from build123d import *

# Parameters (mm, degrees)
SKETCH2_R           = 50
SKETCH2_R_2         = 2
BOSS_EXTRUDE1_DEPTH = 10
SKETCH3_R           = 21.25
SKETCH3_R_2         = 1.75
SKETCH3_R_3         = 10
CUT_EXTRUDE1_DEPTH  = 5
SKETCH3_2_R         = 1.75
CUT_EXTRUDE2_DEPTH  = 75.1479844
SKETCH3_3_R         = 10
CUT_EXTRUDE3_DEPTH  = 75.1479844


with BuildPart() as part:
    # Sketch2 → Boss-Extrude1 (new body)
    # profile 1 of 5: a face of its own
    with BuildSketch(Plane.XY):
        Circle(SKETCH2_R)
        with BuildLine():
            ThreePointArc((-21.767766953, 18.232233047), (-18.232233047, 18.232233047), (-18.232233047, 21.767766953))
            Line((-18.232233047, 21.767766953), (-28.838834765, 32.374368671))
            ThreePointArc((-28.838834765, 32.374368671), (-32.374368671, 32.374368671), (-32.374368671, 28.838834765))
            Line((-32.374368671, 28.838834765), (-21.767766953, 18.232233047))
        make_face(mode=Mode.SUBTRACT)
        with BuildLine():
            ThreePointArc((-18.232233047, -21.767766953), (-18.232233047, -18.232233047), (-21.767766953, -18.232233047))
            Line((-21.767766953, -18.232233047), (-32.374368671, -28.838834765))
            ThreePointArc((-32.374368671, -28.838834765), (-32.374368671, -32.374368671), (-28.838834765, -32.374368671))
            Line((-28.838834765, -32.374368671), (-18.232233047, -21.767766953))
        make_face(mode=Mode.SUBTRACT)
        with BuildLine():
            ThreePointArc((21.767766953, -18.232233047), (18.232233047, -18.232233047), (18.232233047, -21.767766953))
            Line((18.232233047, -21.767766953), (28.838834765, -32.374368671))
            ThreePointArc((28.838834765, -32.374368671), (32.374368671, -32.374368671), (32.374368671, -28.838834765))
            Line((32.374368671, -28.838834765), (21.767766953, -18.232233047))
        make_face(mode=Mode.SUBTRACT)
        with BuildLine():
            ThreePointArc((18.232233047, 21.767766953), (18.232233047, 18.232233047), (21.767766953, 18.232233047))
            Line((21.767766953, 18.232233047), (32.374368671, 28.838834765))
            ThreePointArc((32.374368671, 28.838834765), (32.374368671, 32.374368671), (28.838834765, 32.374368671))
            Line((28.838834765, 32.374368671), (18.232233047, 21.767766953))
        make_face(mode=Mode.SUBTRACT)
    # profile 2 of 5: a face of its own
    with BuildSketch(Plane.XY):
        with BuildLine():
            ThreePointArc((-47.439646086, 15.794935239), (-34.307195372, 36.373291653), (-12.996869684, 48.281273579))
            ThreePointArc((-12.996869684, 48.281273579), (-23.927789331, 47.432136683), (-34.423317157, 50.602299686))
            ThreePointArc((-34.423317157, 50.602299686), (-48.929401728, 47.913811427), (-49.865534018, 33.190424757))
            ThreePointArc((-49.865534018, 33.190424757), (-46.616230999, 24.776660442), (-47.439646086, 15.794935239))
        make_face()
        with Locations((-39.951533137, 39.951533137)):
            Circle(SKETCH2_R_2, mode=Mode.SUBTRACT)
    # profile 3 of 5: a face of its own
    with BuildSketch(Plane.XY):
        with BuildLine():
            ThreePointArc((15.794935239, 47.439646086), (36.373291653, 34.307195372), (48.281273579, 12.996869684))
            ThreePointArc((48.281273579, 12.996869684), (47.432136683, 23.927789331), (50.602299686, 34.423317157))
            ThreePointArc((50.602299686, 34.423317157), (47.913811427, 48.929401728), (33.190424757, 49.865534018))
            ThreePointArc((33.190424757, 49.865534018), (24.776660442, 46.616230999), (15.794935239, 47.439646086))
        make_face()
        with Locations((39.951533137, 39.951533137)):
            Circle(SKETCH2_R_2, mode=Mode.SUBTRACT)
    # profile 4 of 5: a face of its own
    with BuildSketch(Plane.XY):
        with BuildLine():
            ThreePointArc((49.865534018, -33.190424757), (46.616230999, -24.776660442), (47.439646086, -15.794935239))
            ThreePointArc((47.439646086, -15.794935239), (34.307195372, -36.373291653), (12.996869684, -48.281273579))
            ThreePointArc((12.996869684, -48.281273579), (23.927789331, -47.432136683), (34.423317157, -50.602299686))
            ThreePointArc((34.423317157, -50.602299686), (48.929401728, -47.913811427), (49.865534018, -33.190424757))
        make_face()
        with Locations((39.951533137, -39.951533137)):
            Circle(SKETCH2_R_2, mode=Mode.SUBTRACT)
    # profile 5 of 5: a face of its own
    with BuildSketch(Plane.XY):
        with BuildLine():
            ThreePointArc((-33.190424757, -49.865534018), (-24.776660442, -46.616230999), (-15.794935239, -47.439646086))
            ThreePointArc((-15.794935239, -47.439646086), (-36.373291653, -34.307195372), (-48.281273579, -12.996869684))
            ThreePointArc((-48.281273579, -12.996869684), (-47.432136683, -23.927789331), (-50.602299686, -34.423317157))
            ThreePointArc((-50.602299686, -34.423317157), (-47.913811427, -48.929401728), (-33.190424757, -49.865534018))
        make_face()
        with Locations((-39.951533137, -39.951533137)):
            Circle(SKETCH2_R_2, mode=Mode.SUBTRACT)
    extrude(amount=BOSS_EXTRUDE1_DEPTH)

    # Sketch3 → Cut-Extrude1 (cut)
    with BuildSketch(Plane.XY.offset(10)):
        Circle(SKETCH3_R)
        with Locations((0, 14.5)):
            Circle(SKETCH3_R_2, mode=Mode.SUBTRACT)
        with Locations((12.557368355, -7.25)):
            Circle(SKETCH3_R_2, mode=Mode.SUBTRACT)
        with Locations((-12.557368355, -7.25)):
            Circle(SKETCH3_R_2, mode=Mode.SUBTRACT)
        Circle(SKETCH3_R_3, mode=Mode.SUBTRACT)
    extrude(amount=-CUT_EXTRUDE1_DEPTH, mode=Mode.SUBTRACT)

    # Sketch3_2 → Cut-Extrude2 (cut, through all)
    with BuildSketch(Plane.XY.offset(10)):
        with Locations((0, 14.5)):
            Circle(SKETCH3_2_R)
        with Locations((12.557368355, -7.25)):
            Circle(SKETCH3_2_R)
        with Locations((-12.557368355, -7.25)):
            Circle(SKETCH3_2_R)
    extrude(amount=-CUT_EXTRUDE2_DEPTH, mode=Mode.SUBTRACT)

    # Sketch3_3 → Cut-Extrude3 (cut, through all)
    with BuildSketch(Plane.XY.offset(10)):
        Circle(SKETCH3_3_R)
    extrude(amount=-CUT_EXTRUDE3_DEPTH, mode=Mode.SUBTRACT)


solid = part.part
Can you work these out from the model? Positions are in its coordinate system, mm. A direction names the side the tool comes from. Give positions to 0.01 mm unless a question says otherwise; leave off trailing zeros. Order: outer loops, then holes, each group sorted by start corner. A loop starts at its lowest first (then second) coordinate and runs counter-clockwise, first axis right, second up. Notation, with made-up numbers: M 88.25,21.5 L 134.25,21.5 A20 cw 134.25,51.5 Z; hole C 4.25,59.25 d8. An arc over 180 degrees is marked long. One line per question, with ' | ' between items.
Item 1: We'd pull the mould along X, two halves only. Please class faces 3 (the face through (23.461, -26.997, 4.93)), 4 (the face through (49.972, -1.665, 4.93)), 5 (the face through (-1, -22, 10)), 6 (the face through (-46.634, 24.903, 4.93)): released by +X, released by -X, zero draft, split by the parting line, or undercut.
Answer block:
face 3: undercut | face 4: released by +X | face 5: zero draft | face 6: released by -X
Item 2: I'm going to push flat-ended pins straight in: pin 1 Ø5 at (x, z) = (-23.5, 6.5) entering from +Y; pin 2 Ø3 at (x, y) = (12.56, -7.25) entering from -Z; pin 3 Ø6.5 at (x, y) = (39.95, 39.95) entering from +Z; pin 4 Ø13 at (x, y) = (10, -1) entering from +Z. Where does each tip first touch, or does it pass through?
Answer block:
pin 1: stops at y = 47.73 | pin 2: passes through | pin 3: stops at z = 10 | pin 4: stops at z = 5
Item 3: Suppose I cut it at C-C, the plane y = -26. Write out the boundary of the cut face in (x, z).
Answer block:
outline: M -47.73,0 L -29.54,0 L -29.54,10 L -47.73,10 Z; M -22.46,0 L 22.46,0 L 22.46,10 L -22.46,10 Z; M 29.54,0 L 46.83,0 L 46.83,10 L 29.54,10 Z
Item 4: Please list where these lines run through material, in increasing order: L1, parallel to Y at x = 27.5, z = 1.25; L2, parallel to Y at x = 41.5, z = 5; L3, parallel to X at y = -21, z = 4.
Answer block:
L1: y = -48.04 to -31.04, -23.96 to 23.96, 31.04 to 47.19 | L2: y = -51.85 to -41.22, -38.69 to 38.69, 41.22 to 51.85 | L3: x = -47.26 to -24.54, -17.71 to 17.71, 24.54 to 46.45
Item 5: Suppose I cut it at D-D, the plane z = 2.5. Give the number of separate pieces and of enclosed holes in the cut face, then the cut area to 3 significant figures.
Answer block:
separate pieces: 1 | enclosed holes: 12 | area: 8,910 mm2
Item 6: Suppose I cut it at A-A, the plane y = 0. Write out the boundary of the cut face in (x, z).
Answer block:
outline: M -50,0 L -10,0 L -10,5 L -21.25,5 L -21.25,10 L -50,10 Z; M 10,0 L 50,0 L 50,10 L 21.25,10 L 21.25,5 L 10,5 Z
Item 7: For faces 1 (the face through (23.61, 27.145, 4.93)), 2 (the face through (-49.972, 1.665, 4.93)), which set-ups out of +Z, -Z, +X, -X, +Y, -Y let a thin tool reach every point of the face, with its end or its side?
Answer block:
face 1: +Z, -Z | face 2: +Z, -Z, -X
Item 8: Suppose I cut it at B-B, the plane x = -20. Write out the boundary of the cut face in (y, z), then the cut area to 3 significant figures.
Answer block:
outline: M -46.53,0 L -23.54,0 L -23.54,10 L -46.53,10 Z; M -17.5,0 L 17.5,0 L 17.5,10 L 7.18,10 L 7.18,5 L -7.18,5 L -7.18,10 L -17.5,10 Z; M 23.54,0 L 47.27,0 L 47.27,10 L 23.54,10 Z | area: 745 mm2
